Geometry check sheet. Reference: the model listing, model coordinates, mm. Face numbers are marked on the shaded views. A direction names the side the tool comes from. Round coordinates to 2 decimals unless told otherwise and drop trailing zeros. Write each loop counter-clockwise with the first axis right and the second up, starting at its lowest first coordinate (ties: lowest second). Pieces come first, ordered by that corner, then holes. Notation, with made-up numbers: (19, 33) - (35, 33) arc R32 ccw to (35, 69) - close; hole circle Ø4 at (-10.5, 8). An arc over 180 degrees is marked (long way). Return JSON: item names as keys, results as strings. Group by question number.
from build123d import *

# Parameters (mm, degrees)
BOSS_EXTRUDE1_DEPTH = 3
CUT_EXTRUDE1_DEPTH  = 70.878465925
BOSS_EXTRUDE2_DEPTH = 7.5
BOSS_EXTRUDE3_START = 2
BOSS_EXTRUDE3_DEPTH = 2
CUT_EXTRUDE2_DEPTH  = 71.215738976
BOSS_EXTRUDE4_DEPTH = 7.5
CUT_EXTRUDE3_DEPTH  = 71.599220959
BOSS_EXTRUDE5_START = 7.5
BOSS_EXTRUDE5_DEPTH = 7.5
SKETCH10_R          = 2.5
BOSS_EXTRUDE6_DEPTH = 3
FILLET2_R           = 1
SKETCH11_R          = 2.75
CUT_EXTRUDE5_DEPTH  = 71.215738976
FILLET3_R           = 1.5
CUT_EXTRUDE6_DEPTH  = 71.215738976
BOSS_EXTRUDE7_DEPTH = 10.5
CHAMFER1_SIZE       = 1
SKETCH14_W          = 4
SKETCH14_H          = 5.009213965
CUT_EXTRUDE7_DEPTH  = 74.75726829
BOSS_EXTRUDE8_DEPTH = 1.5
FILLET4_R           = 1
FILLET5_R           = 4


with BuildPart() as part:
    # Sketch1 → Boss-Extrude1 (new body)
    with BuildSketch(Plane.XY):
        with BuildLine():
            Line((0.633382655, 2.153501028), (4.366617345, 14.846498972))
            ThreePointArc((4.366617345, 14.846498972), (5.447423794, 16.40203007), (7.244713849, 17))
            Line((7.244713849, 17), (45, 17))
            Line((45, 17), (45, -33))
            ThreePointArc((45, -33), (42.071067812, -40.071067812), (35, -43))
            Line((35, -43), (-55, -43))
            Line((-55, -43), (-55, -3))
            ThreePointArc((-55, -3), (-54.121320344, -0.878679656), (-52, 0))
            Line((-52, 0), (-2.244713849, 0))
            ThreePointArc((-2.244713849, 0), (-0.447423794, 0.59796993), (0.633382655, 2.153501028))
        make_face()
    extrude(amount=BOSS_EXTRUDE1_DEPTH)

    # Sketch2 → Cut-Extrude1 (cut, through all)
    with BuildSketch(Plane.XY.offset(3)):
        with BuildLine():
            Line((-7, -16), (15, -16))
            Line((15, -16), (19.209285015, -35.362711067))
            ThreePointArc((19.209285015, -35.362711067), (18.613549878, -37.882569149), (16.277755923, -39))
            Line((16.277755923, -39), (-7, -39))
            ThreePointArc((-7, -39), (-9.121320344, -38.121320344), (-10, -36))
            Line((-10, -36), (-10, -19))
            ThreePointArc((-10, -19), (-9.121320344, -16.878679656), (-7, -16))
        make_face()
    extrude(amount=-CUT_EXTRUDE1_DEPTH, mode=Mode.SUBTRACT)

    # Sketch3 → Boss-Extrude2 (add)
    with BuildSketch(Plane.XY.offset(3)):
        with BuildLine():
            Line((45, -33), (45, 17))
            Line((45, 17), (7.244713849, 17))
            Line((7.244713849, 17), (7.244713849, 14))
            Line((7.244713849, 14), (42, 14))
            Line((42, 14), (42, -33))
            ThreePointArc((42, -33), (39.949747468, -37.949747468), (35, -40))
            Line((35, -40), (18, -40))
            Line((18, -40), (18, -43))
            Line((18, -43), (35, -43))
            ThreePointArc((35, -43), (42.071067812, -40.071067812), (45, -33))
        make_face()
        Polygon((-5, -43), (-55, -43), (-55, -13), (-52, -13), (-52, -40), (-5, -40), align=None)
    extrude(amount=BOSS_EXTRUDE2_DEPTH)

    # Sketch4 → Boss-Extrude3 (add)
    with BuildSketch(Plane.XY.offset(3).offset(BOSS_EXTRUDE3_START)):
        with BuildLine():
            Line((18.223861668, -12), (-7, -12))
            ThreePointArc((-7, -12), (-11.949747468, -14.050252532), (-14, -19))
            Line((-14, -19), (-14, -36))
            ThreePointArc((-14, -36), (-11.949747468, -40.949747468), (-7, -43))
            Line((-7, -43), (16.277755923, -43))
            ThreePointArc((16.277755923, -43), (21.727941817, -40.392661348), (23.11799047, -34.51299249))
            Line((23.11799047, -34.51299249), (18.223861668, -12))
        make_face()
        with BuildLine():
            Line((15, -16), (-7, -16))
            ThreePointArc((-7, -16), (-9.121320344, -16.878679656), (-10, -19))
            Line((-10, -19), (-10, -36))
            ThreePointArc((-10, -36), (-9.121320344, -38.121320344), (-7, -39))
            Line((-7, -39), (16.277755923, -39))
            ThreePointArc((16.277755923, -39), (18.613549878, -37.882569149), (19.209285015, -35.362711067))
            Line((19.209285015, -35.362711067), (15, -16))
        make_face(mode=Mode.SUBTRACT)
    extrude(amount=-BOSS_EXTRUDE3_DEPTH)

    # Sketch5 → Cut-Extrude2 (cut, through all)
    with BuildSketch(Plane.XY.offset(3)):
        Polygon((9.244713849, 11), (14.744713849, -9), (17.244713849, -9), (11.744713849, 11), align=None)
        Polygon((23.012478168, -9), (17.512478168, 11), (15.012478168, 11), (20.512478168, -9), align=None)
        Polygon((28.780242487, -9), (23.280242487, 11), (20.780242487, 11), (26.280242487, -9), align=None)
        Polygon((34.548006805, -9), (29.048006805, 11), (26.548006805, 11), (32.048006805, -9), align=None)
    extrude(amount=-CUT_EXTRUDE2_DEPTH, mode=Mode.SUBTRACT)

    # Sketch6 → Boss-Extrude4 (add)
    with BuildSketch(Plane.XY.offset(3)):
        Polygon((-52, -40), (-46.641016151, -20), (-52, -20), align=None)
    extrude(amount=BOSS_EXTRUDE4_DEPTH)

    # Sketch7 → Cut-Extrude3 (cut, through all)
    with BuildSketch(Plane.XY.offset(10.5)):
        Polygon((-55, -39.605042507), (-55, -23), (-50.55069227, -23), align=None)
    extrude(amount=-CUT_EXTRUDE3_DEPTH, mode=Mode.SUBTRACT)

    # Sketch8 → Boss-Extrude5 (add)
    with BuildSketch(Plane.XY.offset(3).offset(BOSS_EXTRUDE5_START)):
        with BuildLine():
            Line((-10, -40), (-10, -19))
            ThreePointArc((-10, -19), (-9.121320344, -16.878679656), (-7, -16))
            Line((-7, -16), (-5.183058398, -16))
            Line((-5.183058398, -16), (-5.183058398, -11))
            Line((-5.183058398, -11), (-9.927492456, -11))
            ThreePointArc((-9.927492456, -11), (-11.753776743, -11.619939979), (-12.825269934, -13.223542865))
            Line((-12.825269934, -13.223542865), (-20, -40))
            Line((-20, -40), (-10, -40))
        make_face()
    extrude(amount=-BOSS_EXTRUDE5_DEPTH)

    # Sketch10 → Boss-Extrude6 (add)
    with BuildSketch(Plane.XY.offset(3)):
        with Locations(Location((-50, -5, 0), (0, 0, 180))):
            Circle(SKETCH10_R)
    extrude(amount=BOSS_EXTRUDE6_DEPTH)

    # Fillet2
    fillet2_edges = [part.edges().sort_by_distance(p)[0] for p in [
        (-47.5, -5, 6),
    ]]
    fillet(fillet2_edges, radius=FILLET2_R)

    # Sketch11 → Cut-Extrude5 (cut, through all)
    with BuildSketch(Plane.XY.offset(3)):
        with Locations((35, -33)):
            Circle(SKETCH11_R)
    extrude(amount=-CUT_EXTRUDE5_DEPTH, mode=Mode.SUBTRACT)

    # Fillet3
    fillet3_edges = [part.edges().sort_by_distance(p)[0] for p in [
        (45, -8, 0),
        (42.071067812, -40.071067812, 0),
        (-10, -43, 0),
    ]]
    fillet(fillet3_edges, radius=FILLET3_R)

    # Sketch12 → Cut-Extrude6 (cut, through all)
    with BuildSketch(Plane.XY.offset(3)):
        Polygon((-46.551669862, -36), (-22.551669862, -36), (-22.015771477, -34), (-46.015771477, -34), align=None)
        Polygon((-45.257574636, -31.170370869), (-21.257574636, -31.170370869), (-20.721676251, -29.170370869), (-44.721676251, -29.170370869), align=None)
        Polygon((-43.963479411, -26.340741737), (-19.963479411, -26.340741737), (-19.427581026, -24.340741737), (-43.427581026, -24.340741737), align=None)
        Polygon((-42.669384185, -21.511112606), (-18.669384185, -21.511112606), (-18.1334858, -19.511112606), (-42.1334858, -19.511112606), align=None)
    extrude(amount=-CUT_EXTRUDE6_DEPTH, mode=Mode.SUBTRACT)

    # Sketch13 → Boss-Extrude7 (add)
    with BuildSketch(Plane.XY):
        Polygon((-55, -43), (-53.558551653, -48.009213965), (-14.997432238, -48.009213965), (-14.997432238, -45.504606983), (-12.13347642, -43), align=None)
    extrude(amount=BOSS_EXTRUDE7_DEPTH)

    # Chamfer1
    chamfer1_edges = [part.edges().sort_by_distance(p)[0] for p in [
        (-33.56673821, -43, 0),
        (-34.277991946, -48.009213965, 0),
    ]]
    chamfer(chamfer1_edges, length=CHAMFER1_SIZE)

    # Sketch14 → Cut-Extrude7 (cut, through all)
    with BuildSketch(Plane.XY.offset(10.5)):
        with Locations((-47.558551653, -45.504606983)):
            Rectangle(SKETCH14_W, SKETCH14_H)
        with Locations((-39.558551653, -45.504606983)):
            Rectangle(SKETCH14_W, SKETCH14_H)
        with Locations((-31.558551653, -45.504606983)):
            Rectangle(SKETCH14_W, SKETCH14_H)
        with Locations((-23.558551653, -45.504606983)):
            Rectangle(SKETCH14_W, SKETCH14_H)
    extrude(amount=-CUT_EXTRUDE7_DEPTH, mode=Mode.SUBTRACT)

    # Sketch9 → Boss-Extrude8 (add)
    with BuildSketch(Plane.XY.offset(3)):
        with BuildLine():
            Line((-40, -3.5), (10, -3.5))
            ThreePointArc((10, -3.5), (11.5, -5), (10, -6.5))
            Line((10, -6.5), (-40, -6.5))
            ThreePointArc((-40, -6.5), (-41.5, -5), (-40, -3.5))
        make_face()
    extrude(amount=BOSS_EXTRUDE8_DEPTH)

    # Fillet4
    fillet4_edges = [part.edges().sort_by_distance(p)[0] for p in [
        (-41.5, -5, 4.5),
        (-15, -6.5, 4.5),
        (11.5, -5, 4.5),
        (-15, -3.5, 4.5),
    ]]
    fillet(fillet4_edges, radius=FILLET4_R)

    # Fillet5
    fillet5_edges = [part.edges().sort_by_distance(p)[0] for p in [
        (-5.183058398, -11, 6.75),
    ]]
    fillet(fillet5_edges, radius=FILLET5_R)


solid = part.part
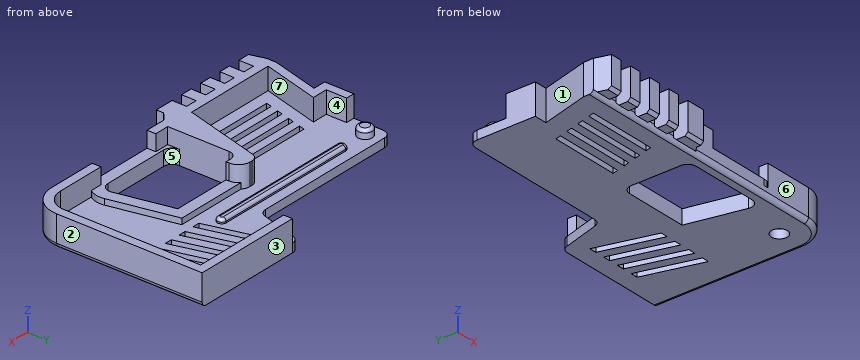
1. Section check B-B (y = 5). Enter the section's corners in (x, z), and give its area (3 significant figures).
2. Section check A-A (x = 3). Enter the section's corners in (y, z).
3. Material ranges on line 1 along Y through (x, z) = (-26.5, 2.5); line 2 along Y through (x, z) = (35, 1.6); line 3 along Z through (x, y) = (-25, -8.5), recorded low to high.
4. Mould release check, pull along X, two halves, no side actions. Record for the marked faces 1, 2, 3 and 4: pulls with the +X half, pulls with the -X half, needs draft (parallel to the pull), parting line crosses it, or undercut.
5. Depth check by flat-ended pin: pin 1 Ø1 at (x, y) = (32.5, -11.5) entering from +Z; pin 2 Ø1.5 at (y, z) = (-35, 8.5) entering from -X; pin 3 Ø3.5 at (y, z) = (16, 5.5) entering from -X; pin 4 Ø8 at (x, y) = (3, -37) entering from -Z. Enter the tip coordinate at first touch or a pass-through.
6. Section check C-C (x = -8). Enter the section's corners in (y, z).
7. Tool access check on the marked faces 5, 6 and 7. Record the directions out of +Z, -Z, +X, -X, +Y, -Y that give a thin tool (end or side, any length) a straight path to the whole face; none if there is none.
Result sheet:
{
 "1": {"outline": "(1.47, 0) - (10.89, 0) - (10.89, 3) - (1.47, 3) - close; (13.39, 0) - (16.66, 0) - (16.66, 3) - (13.39, 3) - close; (19.16, 0) - (22.43, 0) - (22.43, 3) - (19.16, 3) - close; (24.93, 0) - (28.2, 0) - (28.2, 3) - (24.93, 3) - close; (30.7, 0) - (43.5, 0) arc R1.5 ccw to (45, 1.5) - (45, 10.5) - (42, 10.5) - (42, 3) - (30.7, 3) - close", "area": "123 mm²"},
 "2": {"outline": "(-43, 1.5) arc R1.5 ccw to (-41.5, 0) - (-39, 0) - (-39, 5) - (-43, 5) - close; (-16, 0) - (10.2, 0) - (10.2, 3) - (-3.5, 3) - (-3.5, 3.5) arc R1 ccw to (-4.5, 4.5) - (-5.5, 4.5) arc R1 ccw to (-6.5, 3.5) - (-6.5, 3) - (-12, 3) - (-12, 5) - (-16, 5) - close"},
 "3": {"line 1": "y = -48.01 to -36, -34 to -31.17, -29.17 to -26.34, -24.34 to -21.51, -19.51 to 0", "line 2": "y = -43 to -35.75, -30.25 to 17", "line 3": "z = 0 to 3"},
 "4": {"face 1": "pulls with the -X half", "face 2": "pulls with the +X half", "face 3": "needs draft", "face 4": "undercut"},
 "5": {"pin 1": "stops at z = 3", "pin 2": "stops at x = -53.97", "pin 3": "stops at x = 7.24", "pin 4": "stops at z = 0"},
 "6": {"outline": "(-43, 1.5) arc R1.5 ccw to (-41.5, 0) - (-38.83, 0) - (-38.83, 5) - (-40, 5) - (-40, 10.5) - (-43, 10.5) - close; (-16.17, 0) - (0, 0) - (0, 3) - (-3.5, 3) - (-3.5, 3.5) arc R1 ccw to (-4.5, 4.5) - (-5.5, 4.5) arc R1 ccw to (-6.5, 3.5) - (-6.5, 3) - (-11.18, 3) - (-11.18, 10.5) - (-16.17, 10.5) - close"},
 "7": {"face 5": "+Z, -Z", "face 6": "+Z, -Z, +X, -Y", "face 7": "+Z"}
}
